```python
from build123d import *

# Parameters (mm, degrees)
PAD002_DEPTH = 12.5


with BuildPart() as part:
    # Sketch003 → Pad002 (new body, symmetric)
    with BuildSketch(Plane.XZ):
        with BuildLine():
            Line((-22.5, 59.5), (22.5, 59.5))
            Line((22.5, 59.5), (50.596605, 67.5))
            Line((50.596605, 67.5), (87, 67.5))
            ThreePointArc((87.433912, 62.537944), (89.490496, 65.217784), (87, 67.5))
            Line((87.433912, 62.537944), (47.5, 55.5))
            Line((47.5, 55.5), (39.5, 47.5))
            Line((39.5, 47.5), (43.014719, 47.5))
            Line((43.014719, 47.5), (45.5, 45.014719))
            Line((45.5, 45.014719), (45.5, 30.5))
            Line((45.5, 30.5), (47.5, 24.5))
            Line((47.5, 24.5), (42.5, 20.5))
            Line((42.5, 20.5), (26.5, 17.5))
            Line((26.5, 17.5), (22.5, 27.5))
            Line((-22.5, 27.5), (22.5, 27.5))
            Line((-22.5, 27.5), (-26.5, 17.5))
            Line((-26.5, 17.5), (-42.5, 20.5))
            Line((-42.5, 20.5), (-47.5, 24.5))
            Line((-47.5, 24.5), (-45.5, 30.5))
            Line((-45.5, 30.5), (-45.5, 45.014719))
            Line((-45.5, 45.014719), (-43.014719, 47.5))
            Line((-43.014719, 47.5), (-39.5, 47.5))
            Line((-39.5, 47.5), (-47.5, 55.5))
            Line((-47.5, 55.5), (-87.433912, 62.537944))
            ThreePointArc((-87, 67.5), (-89.490496, 65.217784), (-87.433912, 62.537944))
            Line((-87, 67.5), (-50.596605, 67.5))
            Line((-50.596605, 67.5), (-22.5, 59.5))
        make_face()
    extrude(amount=PAD002_DEPTH, both=True)


solid = part.part
```
Work out the finished part from the listing and answer in its coordinate system (mm). A direction names the side the tool comes from. Give positions to 0.01 mm unless a question says otherwise; leave off trailing zeros. Loops run counter-clockwise (first coordinate to the right, second up) from the corner with the lowest first, then second, coordinate; pieces in that order, holes last. Notation, with made-up numbers: M 80.25,-2 L 119.25,-2 A19 cw 119.25,26 Z; hole C -39.75,19.5 d5. An arc over 180 degrees is marked long. One line per item, written item: value. Start each with the question number.
1. Find the intervals of material crossed by probe 1 along X at (y, z) = (11.5, 44); probe 2 along X at (y, z) = (-3, 23) (3 decimals); probe 3 along Z at (x, y) = (15, -11.25), in increasing order.
2. Each of these flat-tipped pins is pushed along its axis until it touches: P1, Ø1, axis at x = 9, y = -5.5, coming from the +Z side; P2, Ø1.1, axis at x = 41, y = 6, coming from the +Z side; P3, Ø1.1, axis at x = -41.5, y = 4, coming from the +Z side. Where does it stop, or does it pass through?
3. Find section B-B (x = -20.5). Give the vertices of the cut face in (y, z).
4. Determine the mould class of faces 4 (the face through (-34.39, -0.18, 18.98)), 5 (the face through (0, 0, 59.5)), 6 (the face through (67.75, -0.18, 59.07)) for opening direction X: released by +X, released by -X, zero draft, split by the parting line, or undercut.
5. Find section A-A (y = 3.5). Give the vertices of the cut face in (x, z).
6. Find section C-C (z = 35.5). Give the vertices of the cut face in (x, y).
7. Which of the six approach directions +Z, -Z, +X, -X, +Y, -Y give full straight-line access (tool end or side, diameter ignored) to faces 1 (the face through (-45.5, 0, 38)), 2 (the face through (0, 0, 27.5)), 3 (the face through (45.5, 0, 38))?
Reported:
1. probe 1: x = -45.5 to 45.5
1. probe 2: x = -45.625 to -24.3, 24.3 to 45.625
1. probe 3: z = 27.5 to 59.5
2. P1: stops at z = 59.5
2. P2: stops at z = 64.92
2. P3: stops at z = 65.07
3. outline: M -12.5,27.5 L 12.5,27.5 L 12.5,59.5 L -12.5,59.5 Z
4. face 4: released by -X
4. face 5: undercut
4. face 6: released by +X
5. outline: M -87.43,62.54 L -47.5,55.5 L -39.5,47.5 L -43.01,47.5 L -45.5,45.01 L -45.5,30.5 L -47.5,24.5 L -42.5,20.5 L -26.5,17.5 L -22.5,27.5 L 22.5,27.5 L 26.5,17.5 L 42.5,20.5 L 47.5,24.5 L 45.5,30.5 L 45.5,45.01 L 43.01,47.5 L 39.5,47.5 L 47.5,55.5 L 87.43,62.54 A2.5 ccw 87,67.5 L 50.6,67.5 L 22.5,59.5 L -22.5,59.5 L -50.6,67.5 L -87,67.5 A2.5 ccw Z
6. outline: M -45.5,-12.5 L 45.5,-12.5 L 45.5,12.5 L -45.5,12.5 Z
7. face 1: -X, +Y, -Y
7. face 2: -Z, +Y, -Y
7. face 3: +X, +Y, -Y
